Verification items for this drawing (mm, ordinates from the low corner). A direction names the side the tool comes from. Coordinates: 2 decimals unless noted, no trailing zeros. Loops run counter-clockwise (first coordinate to the right, second up) from the corner with the lowest first, then second, coordinate; pieces in that order, holes last. Notation, with made-up numbers: (74.5, 25.5) - (115.5, 25.5) arc R17 ccw to (115.5, 30.5) - close; hole circle Ø6 at (22.25, 66). An arc over 180 degrees is marked (long way). One line per item, written item: value. Start each with the question number.
(1) Section check B-B (z = 2.5). Record the boundary of the cut face in (x, y), plus the area to 3 significant figures.
(2) Gauge pin test, flat ends, axial feed: P1, Ø3, axis at x = 14, y = 17.5, coming from the +Z side; P2, Ø7, axis at x = 10, z = 10, coming from the +Y side; P3, Ø5, axis at x = 12.5, z = 10.5, coming from the +Y side. Record the tip position at first contact, or that the pin passes through.
(3) Section check A-A (y = 13). Record the boundary of the cut face in (x, z), plus the area to 3 significant figures.
(4) Set-up check for the marked faces 1 and 2: record each of +Z, -Z, +X, -X, +Y, -Y from which the full face is reachable in a straight line by a thin tool's end or side.
(5) Draft check along X on the marked faces 3, 4 and 5. Enter one of: +X half, -X half, draft (parallel to the pull), parting line (faces both ways), or undercut.
(6) Section check D-D (x = 3). Record the boundary of the cut face in (y, z), plus the area to 3 significant figures.
(7) Thickness scan on probe 1 along Y at (x, z) = (10, 0.8); probe 2 along Y at (x, z) = (14.75, 17.75). Record the ranges inside material, lowest first. Write a range as [from, to].
(8) Section check C-C (y = 7.25). Record the boundary of the cut face in (x, z).
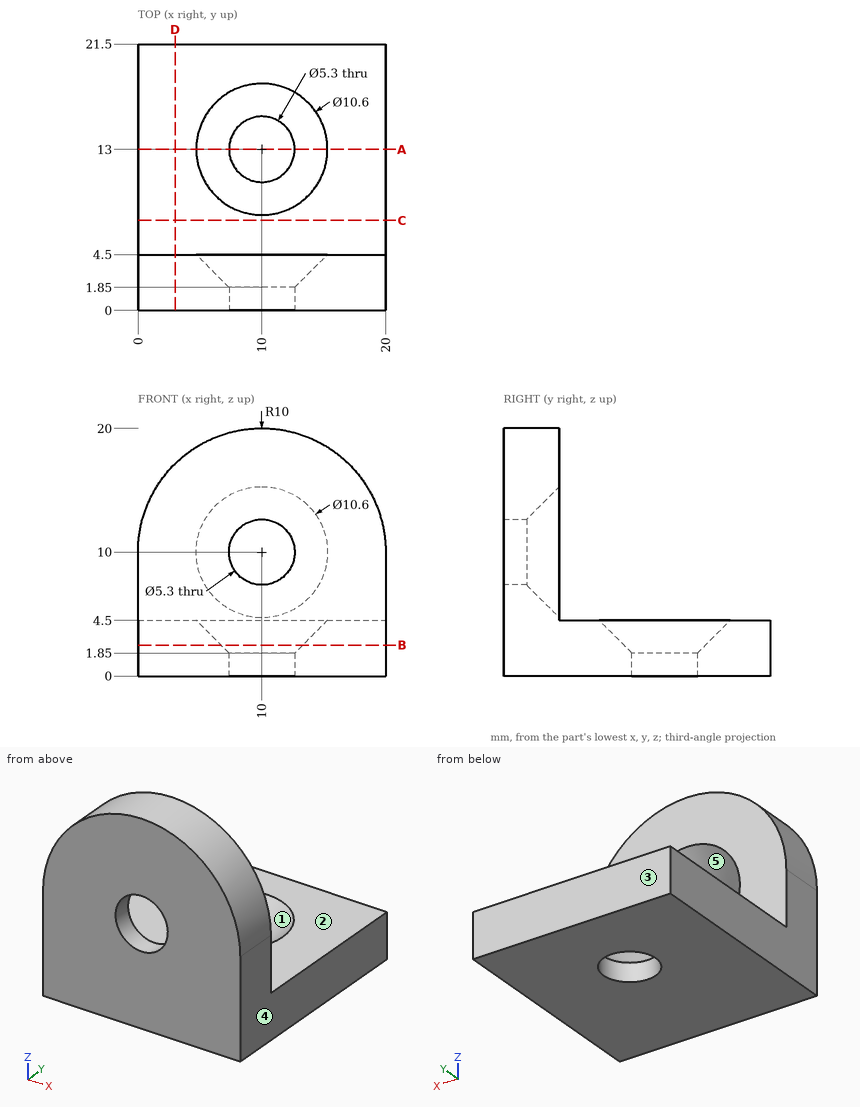
Responses:
1. outline: (0, 0) - (20, 0) - (20, 21.5) - (0, 21.5) - close; hole circle Ø6.6 at (10, 13)
1. area: 396 mm²
2. P1: stops at z = 4.5
2. P2: stops at y = 2.7
2. P3: stops at y = 4.25
3. outline: (0, 0) - (7.35, 0) - (7.35, 1.85) - (4.7, 4.5) - (0, 4.5) - close; (12.65, 0) - (20, 0) - (20, 4.5) - (15.3, 4.5) - (12.65, 1.85) - close
3. area: 59.1 mm²
4. face 1: +Z
4. face 2: +Z, +X, -X, +Y
5. face 3: draft
5. face 4: +X half
5. face 5: undercut
6. outline: (0, 0) - (21.5, 0) - (21.5, 4.5) - (4.5, 4.5) - (4.5, 17.14) - (0, 17.14) - close
6. area: 154 mm²
7. probe 1: y = [0, 10.35], [15.65, 21.5]
7. probe 2: y = [0, 4.5]
8. outline: (0, 0) - (20, 0) - (20, 4.5) - (0, 4.5) - close
